Geometry: final body of the model. Coordinates: model frame, mm. A direction names the side the tool comes from. Give positions to 0.01 mm unless a question says otherwise; leave off trailing zeros. Write each loop counter-clockwise with the first axis right and the second up, starting at its lowest first coordinate (ties: lowest second). Pieces come first, ordered by that corner, then holes.
from build123d import *

# Parameters (mm, degrees)
F0_W     = 25.4
F0_H     = 76.2
F1_DEPTH = 7.62
F2_R     = 6.35
F3_DEPTH = 5.08
F4_R     = 3.81
F5_DEPTH = 5.08


with BuildPart() as f1:
    # F0 (on Top) → F1 (new body)
    with BuildSketch(Plane.XY):
        with Locations((-3.308222, 10.889477)):
            Rectangle(F0_W, F0_H)
    extrude(amount=F1_DEPTH)

    # F2 (on face) → F3 (cut)
    with BuildSketch(Plane(origin=(0, 0, 0), x_dir=(1, 0, 0), z_dir=(0, 0, -1))):
        with Locations((-3.308222, 14.510523)):
            Circle(F2_R)
    extrude(amount=-F3_DEPTH, mode=Mode.SUBTRACT)

    # F4 (on face) → F5 (cut)
    with BuildSketch(Plane(origin=(0, 0, 0), x_dir=(1, 0, 0), z_dir=(0, 0, -1))):
        with Locations((-9.658222, -42.639477)):
            Circle(F4_R)
    extrude(amount=-F5_DEPTH, mode=Mode.SUBTRACT)


solid = f1.part
Q1. Section C-C on x = -8.5. Output: boundary loops of the cut face in (y, z), plus the area to 3 significant figures.
Filled sheet:
outline: (-27.21, 0) - (-18.17, 0) - (-18.17, 5.08) - (-10.85, 5.08) - (-10.85, 0) - (39.01, 0) - (39.01, 5.08) - (46.27, 5.08) - (46.27, 0) - (48.99, 0) - (48.99, 7.62) - (-27.21, 7.62) - close
area: 507 mm2
Q2. Access query for faces 5 (the flat face through (-3, 11, 7.62)), 6 (the flat face through (-10, 43, 5.08)). Directions: +Z, -Z, +X, -X, +Y, -Y. A direction counts if a zero-diameter tool reaches every point of the face in a straight line with its end or side. Return the directions, or none.
Filled sheet:
face 5: +Z, +X, -X, +Y, -Y
face 6: -Z
Q3. Pull-direction query (X, two-part tool) for faces 1 (the flat face through (9.392, 10, 4)), 2 (the cylindrical face through (-4.68, -8.31, 2.5)), 3 (the flat face through (-3, 11, 0)), 4 (the flat face through (-16.008, 10, 4)); classes: released by +X, released by -X, zero draft, split by the parting line, or undercut.
Filled sheet:
face 1: released by +X
face 2: undercut
face 3: zero draft
face 4: released by -X
Q4. Pin query (flat end, axial travel): P1, Ø7.5, axis at x = -3.31, y = -14.51, coming from the -Z side. Return the tip coordinate at first contact, or that it passes through.
Filled sheet:
P1: stops at z = 5.08
Q5. Ray query, line 1 along X through (y, z) = (-15.5, 2.25); line 2 along X through (y, z) = (-12, 0.75); line 3 along Y through (x, z) = (-12.25, 5). Return the intervals inside material, ascending.
Filled sheet:
line 1: x = -16.01 to -9.58, 2.96 to 9.39
line 2: x = -16.01 to -9.14, 2.52 to 9.39
line 3: y = -27.21 to 39.85, 45.43 to 48.99
Q6. Section B-B on z = 2.5. Output: boundary loops of the cut face in (x, y), plus the area to 3 significant figures.
Filled sheet:
outline: (-16.01, -27.21) - (9.39, -27.21) - (9.39, 48.99) - (-16.01, 48.99) - close; hole circle Ø7.62 at (-9.66, 42.64); hole circle Ø12.7 at (-3.31, -14.51)
area: 1,760 mm2
Q7. Section A-A on x = -4.25. Output: boundary loops of the cut face in (y, z).
Filled sheet:
outline: (-27.21, 0) - (-20.79, 0) - (-20.79, 5.08) - (-8.23, 5.08) - (-8.23, 0) - (48.99, 0) - (48.99, 7.62) - (-27.21, 7.62) - close
